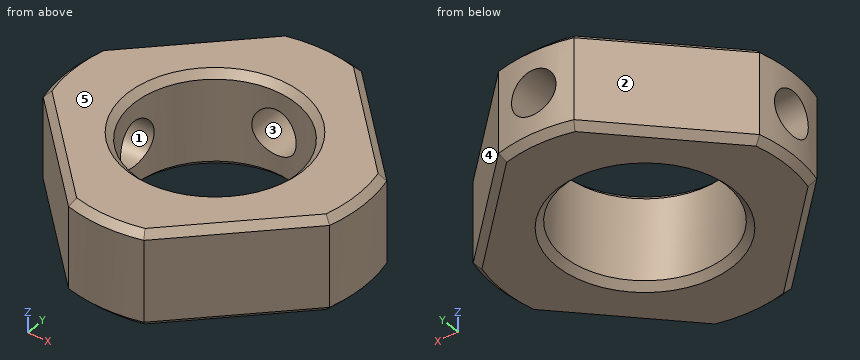
```python
from build123d import *

# Parameters (mm, degrees)
SKETCH1_R           = 6
BOSS_EXTRUDE1_DEPTH = 3.5
SKETCH2_OUTSIDE_W   = 36.598
SKETCH2_OUTSIDE_H   = 36.598
SKETCH2_OUTSIDE_R   = 11
CUT_EXTRUDE1_DEPTH  = 8
SKETCH4_R           = 1.65
CUT_EXTRUDE2_DEPTH  = 12
SKETCH5_R           = 1.65
CUT_EXTRUDE3_DEPTH  = 12
CHAMFER1_SIZE       = 0.5


with BuildPart() as part:
    # Sketch1 → Boss-Extrude1 (new body, symmetric)
    with BuildSketch(Plane.XY):
        Polygon((0, -13.435028843), (-13.435028843, 0), (0, 13.435028843), (13.435028843, 0), align=None)
        Circle(SKETCH1_R, mode=Mode.SUBTRACT)
    extrude(amount=BOSS_EXTRUDE1_DEPTH, both=True)

    # Sketch2 outside → Cut-Extrude1 (cut, through all)
    with BuildSketch(Plane.XY.offset(3.5)):
        Rectangle(SKETCH2_OUTSIDE_W, SKETCH2_OUTSIDE_H)
        Circle(SKETCH2_OUTSIDE_R, mode=Mode.SUBTRACT)
    extrude(amount=-CUT_EXTRUDE1_DEPTH, mode=Mode.SUBTRACT)

    # Sketch4 → Cut-Extrude2 (cut, through all)
    with BuildSketch(Plane(origin=(0, 0, 0), x_dir=(1, 0, 0), z_dir=(0, 1, 0))):
        Circle(SKETCH4_R)
    extrude(amount=CUT_EXTRUDE2_DEPTH, mode=Mode.SUBTRACT)

    # Sketch5 → Cut-Extrude3 (cut, through all)
    with BuildSketch(Plane(origin=(0, 0, 0), x_dir=(0, 0, -1), z_dir=(1, 0, 0))):
        Circle(SKETCH5_R)
    extrude(amount=-CUT_EXTRUDE3_DEPTH, mode=Mode.SUBTRACT)

    # Chamfer1
    chamfer1_edges = [part.edges().sort_by_distance(p)[0] for p in [
        (-6, 0, -3.5),
        (-6, 0, 3.5),
        (6.717514421, 6.717514421, -3.5),
        (6.717514421, 6.717514421, 3.5),
        (6.717514421, -6.717514421, -3.5),
        (6.717514421, -6.717514421, 3.5),
        (-6.717514421, -6.717514421, -3.5),
        (-6.717514421, -6.717514421, 3.5),
        (-6.717514421, 6.717514421, -3.5),
        (-6.717514421, 6.717514421, 3.5),
        (-11, 0, -3.5),
        (0, -11, -3.5),
        (11, 0, -3.5),
        (0, 11, -3.5),
        (0, 11, 3.5),
        (-11, 0, 3.5),
        (0, -11, 3.5),
        (11, 0, 3.5),
    ]]
    chamfer(chamfer1_edges, length=CHAMFER1_SIZE)


solid = part.part
```
Can you work these out from the model? Positions are in its coordinate system, mm. Face numbers are marked on the shaded views. A direction names the side the tool comes from. Give positions to 0.01 mm unless a question says otherwise; leave off trailing zeros. Write each loop counter-clockwise with the first axis right and the second up, starting at its lowest first coordinate (ties: lowest second). Pieces come first, ordered by that corner, then holes. Notation, with made-up numbers: (7.25, -11) - (40.25, -11) arc R26 ccw to (40.25, 20) - close; hole circle Ø2 at (60, 47.25). An arc over 180 degrees is marked (long way). Write item = value, one per line. Start each with the question number.
1. Imagine slicing it at B-B (x = 0). Please give me the cut outline in (y, z).
2. Imagine slicing it at D-D (x = 7.25). Please give me the cut outline in (y, z), and give its area (3 significant figures).
3. On a 3-axis mill with a long thin cutter (end or side, diameter ignored), from which of +Z, -Z, +X, -X, +Y, -Y can I reach the whole of each face in a straight line? I mean the marked faces 1 and 2. Say none if no direction works.
4. Imagine slicing it at A-A (y = 0). Please give me the cut outline in (x, z).
5. Imagine slicing it at C-C (z = 0). Please give me the cut outline in (x, y), and give its area (3 significant figures).
6. For pin 1 (2.5 mm diameter, centred on x = 0, z = 0, fed in from +Y); pin 2 (7 mm diameter, centred on x = 0, y = 0, fed in from +Z); pin 3 (2 mm diameter, centred on y = 6.5, z = -2.5, fed in from +X) (3 decimals); pin 4 (2 mm diameter, centred on y = -5, z = 1.5, fed in from -X) (3 decimals), each with a flat end and sliding along its axis, tell me the tip position at first contact or that it passes through.
7. Thinking about a two-plate mould opening in Z: for the marked faces 3, 4 and 5, which applies, released by +Z, released by -Z, zero draft, split by the parting line, or undercut?
8. Please list where these lines run through material, in increasing order: line 1 (X direction, y = -0.25, z = -1.75); line 2 (Z direction, x = -7.25, y = 0); line 3 (Y direction, x = 3.25, z = -1.25).
Worked answers:
q1.outline = (-11, -3) - (-10.5, -3.5) - (-6.5, -3.5) - (-6, -3) - (-6, 3) - (-6.5, 3.5) - (-10.5, 3.5) - (-11, 3) - close; (6, -3) - (6.5, -3.5) - (10.5, -3.5) - (11, -3) - (11, -1.65) - (6, -1.65) - close; (6, 1.65) - (11, 1.65) - (11, 3) - (10.5, 3.5) - (6.5, 3.5) - (6, 3) - close
q2.outline = (-6.19, -3) - (-5.48, -3.5) - (5.48, -3.5) - (6.19, -3) - (6.19, 3) - (5.48, 3.5) - (-5.48, 3.5) - (-6.19, 3) - close
q2.area = 85.9 mm2
q3.face_1 = -X
q3.face_2 = +Z, -Z, -X, +Y
q4.outline = (-11, -3) - (-10.5, -3.5) - (-6.5, -3.5) - (-6, -3) - (-6, -1.65) - (-11, -1.65) - close; (-11, 1.65) - (-6, 1.65) - (-6, 3) - (-6.5, 3.5) - (-10.5, 3.5) - (-11, 3) - close; (6, -3) - (6.5, -3.5) - (10.5, -3.5) - (11, -3) - (11, 3) - (10.5, 3.5) - (6.5, 3.5) - (6, 3) - close
q5.outline = (-10.88, -1.65) arc R11 ccw to (-10.64, -2.8) - (-2.8, -10.64) arc R11 ccw to (2.8, -10.64) - (10.64, -2.8) arc R11 ccw to (10.64, 2.8) - (2.8, 10.64) arc R11 ccw to (1.65, 10.88) - (1.65, 5.77) arc R6 cw (long way) to (-5.77, -1.65) - close; (-10.88, 1.65) - (-5.77, 1.65) arc R6 cw to (-1.65, 5.77) - (-1.65, 10.88) arc R11 ccw to (-2.8, 10.64) - (-10.64, 2.8) arc R11 ccw to start
q5.area = 189 mm2
q6.pin_1 = -5.87
q6.pin_2 = through
q6.pin_3 = 7.935
q6.pin_4 = -9.435
q7.face_3 = undercut
q7.face_4 = zero draft
q7.face_5 = released by +Z
q8.line_1 = -11 to -5.99, 5.99 to 11
q8.line_2 = -3.5 to -1.65, 1.65 to 3.5
q8.line_3 = -10.19 to -5.04, 5.04 to 10.19
